```python
from build123d import *

# Parameters (mm, degrees)
ESQUISSE2_R             = 1.5
ENL_V_MAT_EXTRU_1_DEPTH = 139.855140344
CUT_EXTRUDE4_DEPTH      = 142.779758781
CUT_EXTRUDE4_DEPTH_BACK = 16.77
SKETCH6_R               = 54.5
SKETCH6_R_2             = 53.5
CUT_EXTRUDE5_DEPTH      = 136.957714014
CUT_EXTRUDE5_DEPTH_BACK = 136.957714014
SKETCH7_R               = 1.5
CUT_EXTRUDE6_DEPTH      = 136.957714098
CUT_EXTRUDE6_DEPTH_BACK = 136.957714098
SKETCH8_R               = 1.5


with BuildPart() as part:
    # Esquisse1 → Base-Révolution (revolve)
    with BuildSketch(Plane(origin=(0, 0, 0), x_dir=(0, 0, -1), z_dir=(1, 0, 0)), mode=Mode.PRIVATE) as base_r_volution_sk:
        with BuildLine():
            Line((112, 34.4), (112, 42.5))
            Line((112, 42.5), (111, 42.5))
            ThreePointArc((111, 42.5), (105.301147892, 51.14939936), (95.5, 54.5))
            Line((95.5, 54.5), (-7, 54.5))
            Line((-7, 54.5), (-7, 53.5))
            Line((-7, 53.5), (93.35, 53.5))
            ThreePointArc((93.35, 53.5), (102.082768748, 49.882768748), (105.7, 41.15))
            Line((105.7, 41.15), (108.5, 41.15))
            Line((108.5, 41.15), (108.5, 35.5))
            Line((108.5, 35.5), (110, 35.5))
            Line((110, 35.5), (110, 34.4))
            Line((110, 34.4), (112, 34.4))
        make_face()
    revolve(base_r_volution_sk.sketch.rotate(Axis((0, 0, 74.926735219), (0, 0, -1)), 90), axis=Axis((0, 0, 74.926735219), (0, 0, -1)))

    # Esquisse2 → Enlèv. mat.-Extru.1 (cut, through all)
    with BuildSketch(Plane.XY.offset(-108.5)):
        with Locations((0, 38)):
            Circle(ESQUISSE2_R)
        with Locations((19, 32.908965344)):
            Circle(ESQUISSE2_R)
        with Locations((32.908965344, 19)):
            Circle(ESQUISSE2_R)
        with Locations((38, 0)):
            Circle(ESQUISSE2_R)
        with Locations((32.908965344, -19)):
            Circle(ESQUISSE2_R)
        with Locations((19, -32.908965344)):
            Circle(ESQUISSE2_R)
        with Locations((0, -38)):
            Circle(ESQUISSE2_R)
        with Locations((-19, -32.908965344)):
            Circle(ESQUISSE2_R)
        with Locations((-32.908965344, -19)):
            Circle(ESQUISSE2_R)
        with Locations((-38, 0)):
            Circle(ESQUISSE2_R)
        with Locations((-32.908965344, 19)):
            Circle(ESQUISSE2_R)
        with Locations((-19, 32.908965344)):
            Circle(ESQUISSE2_R)
    extrude(amount=-ENL_V_MAT_EXTRU_1_DEPTH, mode=Mode.SUBTRACT)

    # Sketch6 → Cut-Extrude4 (cut, two sides: drawn at the far end of the back side and taken through both)
    with BuildSketch(Plane.XY.offset(7).offset(-CUT_EXTRUDE4_DEPTH_BACK)):
        Circle(SKETCH6_R)
        Circle(SKETCH6_R_2, mode=Mode.SUBTRACT)
    extrude(amount=CUT_EXTRUDE4_DEPTH + CUT_EXTRUDE4_DEPTH_BACK, mode=Mode.SUBTRACT)

    # Sketch7 → Cut-Extrude5 (cut, two sides: drawn at the far end of the back side and taken through both)
    with BuildSketch(Plane(origin=(0, 0, 0), x_dir=(1, 0, 0), z_dir=(0, 1, 0)).offset(-CUT_EXTRUDE5_DEPTH_BACK)):
        with Locations(Location((0, 19.86, 0), (0, 0, 270))):
            Circle(SKETCH7_R)
    extrude(amount=CUT_EXTRUDE5_DEPTH + CUT_EXTRUDE5_DEPTH_BACK, mode=Mode.SUBTRACT)

    # Sketch8 → Cut-Extrude6 (cut, two sides: drawn at the far end of the back side and taken through both)
    with BuildSketch(Plane(origin=(0, 0, 0), x_dir=(0, 0, -1), z_dir=(1, 0, 0)).offset(-CUT_EXTRUDE6_DEPTH_BACK)):
        with Locations((19.86, 0)):
            Circle(SKETCH8_R)
    extrude(amount=CUT_EXTRUDE6_DEPTH + CUT_EXTRUDE6_DEPTH_BACK, mode=Mode.SUBTRACT)


solid = part.part
```
The listing builds one solid part. Answer for the finished solid, in the listing's coordinates (mm). A direction names the side the tool comes from. Round coordinates to 2 decimals unless told otherwise and drop trailing zeros. Order: outer loops, then holes, each group sorted by start corner. A loop starts at its lowest first (then second) coordinate and runs counter-clockwise, first axis right, second up. Notation, with made-up numbers: (60.25, 60.5) -> (65.25, 60.5) arc R8 cw to (65.25, 69.5) -> close; hole circle Ø10 at (62, -9). An arc over 180 degrees is marked (long way). Answer as CSV lines item,"result".
Q1. A cutting plane is placed at B-B on y = 0. Give the number of separate pieces and of enclosed holes in the cut face, plus the area to 3 significant figures.
Computed values:
separate pieces,"6"
enclosed holes,"0"
area,"322 mm^2"
Q2. Which of the six approach directions +Z, -Z, +X, -X, +Y, -Y give full straight-line access (tool end or side, diameter ignored) to faces 1 (the cylindrical face through (-34.015, 20.014, -110.226)), 2 (the flat face through (-31, -18, -108.5))?
Computed values:
face 1,"+Z, -Z"
face 2,"+Z"
Q3. For a pull along Y with two mould halves and no side action, classify faces 3 (the cylindrical face through (-39.2, -0.9, -110.2)), 4 (the flat face through (40, -36, -9.77)), 5 (the cylindrical face through (40.537, -12.766, -111.493)) as +Y half, -Y half, draft (parallel to the pull), parting line (faces both ways), or undercut.
Computed values:
face 3,"undercut"
face 4,"draft"
face 5,"parting line"
Q4. A cutting plane is placed at A-A on z = -91.5. Determine the outline of the cut face in (x, y).
Computed values:
outline,"circle Ø109 at (0, 0); hole circle Ø107 at (0, 0)"
Q5. Given pin 1 (12 mm diameter, centred on y = -28.5, z = -87, fed in from +X); pin 2 (5 mm diameter, centred on x = -32.91, y = 19, fed in from +Z); pin 3 (3 mm diameter, centred on y = 25, z = -24, fed in from +X), each flat-ended and moving along its own axis, determine where each tip first touches the part or whether it passes through.
Computed values:
pin 1,"stops at x = 49.64"
pin 2,"stops at z = -108.5"
pin 3,"stops at x = 49.17"
Q6. Consider line 1 (Y direction, x = -19, z = -109); line 2 (Y direction, x = 0, z = -69.5); line 3 (X direction, y = -5, z = -14). Determine where each line is inside the solid, lowest interval first. Write a range as from..to.
Computed values:
line 1,"y = -43.09..-34.41, -31.41..-29.99, 29.99..31.41, 34.41..43.09"
line 2,"y = -54.5..-53.5, 53.5..54.5"
line 3,"x = -54.27..-53.27, 53.27..54.27"
